Study the drawing (mm; zero at the part's minimum x, y, z) and answer. Coordinates: 2 decimals unless noted, no trailing zeros. Loops run counter-clockwise (first coordinate to the right, second up) from the corner with the lowest first, then second, coordinate; pieces in that order, holes last. Notation, with made-up numbers: (27.5, 24) - (62.5, 24) arc R4 cw to (62.5, 28) - close; hole circle Ø7 at (50, -5). An arc over 180 degrees is marked (long way). Use one line per item in the form item = value.
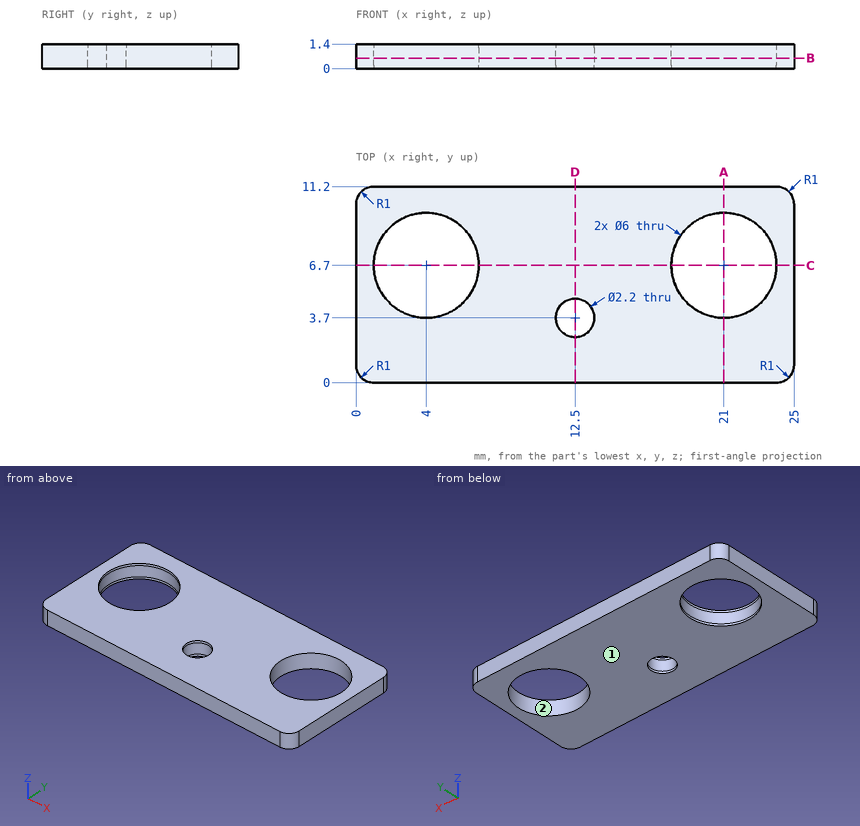
Item 1: The part is cut by section D-D on x = 12.5. Give the vertices of the cut face in (y, z).
Results below:
outline = (0, 0) - (2.6, 0) - (2.6, 1.4) - (0, 1.4) - close; (4.8, 0) - (11.2, 0) - (11.2, 1.4) - (4.8, 1.4) - close
Item 2: The part is cut by section C-C on y = 6.7. Give the vertices of the cut face in (x, z), plus the area to 3 significant figures.
Results below:
outline = (0, 0) - (1, 0) - (1, 1.4) - (0, 1.4) - close; (7, 0) - (18, 0) - (18, 1.4) - (7, 1.4) - close; (24, 0) - (25, 0) - (25, 1.4) - (24, 1.4) - close
area = 18.2 mm²
Item 3: This flat-tipped pin is pushed along its axis until it touches: P1, Ø2.5, axis at x = 12.5, y = 3.7, coming from the +Z side. Where does it stop, or does it pass through?
Results below:
P1 = 1.4
Item 4: For a pull along X with two mould halves and no side action, classify the marked faces 1 and 2 as +X half, -X half, draft (parallel to the pull), parting line (faces both ways), or undercut.
Results below:
face_1 = draft
face_2 = undercut
Item 5: The part is cut by section A-A on x = 21. Give the vertices of the cut face in (y, z).
Results below:
outline = (0, 0) - (3.7, 0) - (3.7, 1.4) - (0, 1.4) - close; (9.7, 0) - (11.2, 0) - (11.2, 1.4) - (9.7, 1.4) - close
Item 6: Find the intervals of material crossed by L1, parallel to X at y = 6.7, z = 0.5; L2, parallel to Y at x = 4, z = 0.55; L3, parallel to Y at x = 12.5, z = 0.85, in increasing order.
Results below:
L1 = 0 to 1, 7 to 18, 24 to 25
L2 = 0 to 3.7, 9.7 to 11.2
L3 = 0 to 2.6, 4.8 to 11.2
Item 7: The part is cut by section B-B on z = 0.6. Give the vertices of the cut face in (x, y).
Results below:
outline = (0, 1) arc R1 ccw to (1, 0) - (24, 0) arc R1 ccw to (25, 1) - (25, 10.2) arc R1 ccw to (24, 11.2) - (1, 11.2) arc R1 ccw to (0, 10.2) - close; hole circle Ø6 at (4, 6.7); hole circle Ø2.2 at (12.5, 3.7); hole circle Ø6 at (21, 6.7)
